CAD build for the part. Positions are in the model's coordinates, mm. Face numbers are marked on the shaded views. Coordinates: 2 decimals unless noted, no trailing zeros. Order: outer loops, then holes, each group sorted by start corner. A loop starts at its lowest first (then second) coordinate and runs counter-clockwise, first axis right, second up. Notation, with made-up numbers: M 3,23.5 L 35,23.5 A32 ccw 35,50.5 Z; hole C 77,42 d8. An arc over 180 degrees is marked long. Write item = value, one per line.
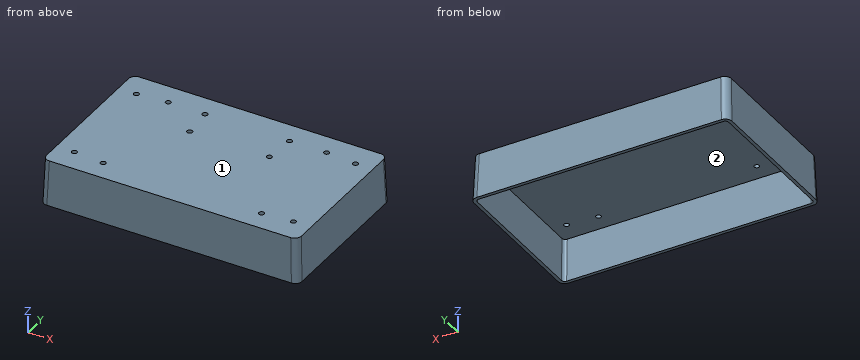
from build123d import *

# Parameters (mm, degrees)
SKETCH_1_W      = 148
SKETCH_1_H      = 88
SKETCH_1_R      = 1.5
EXTRUDE_1_DEPTH = 25
EXTRUDE_1_DRAFT = 2
FILLET_1_R      = 2
SHELL_1_T       = 2


with BuildPart() as part:
    # Эскиз1 → Бобышка-Вытянуть1 (with draft: the straight prism first)
    with BuildSketch(Plane.XY):
        with Locations((-40.018678, 18.487832)):
            Rectangle(SKETCH_1_W, SKETCH_1_H)
        with Locations((7.364962, 51.289097)):
            Circle(SKETCH_1_R, mode=Mode.SUBTRACT)
        with Locations((25.491262, 49.776217)):
            Circle(SKETCH_1_R, mode=Mode.SUBTRACT)
        with Locations((25.471663, -13.623467)):
            Circle(SKETCH_1_R, mode=Mode.SUBTRACT)
        with Locations((7.364962, -15.128048)):
            Circle(SKETCH_1_R, mode=Mode.SUBTRACT)
        with Locations((-14.633582, 51.078679)):
            Circle(SKETCH_1_R, mode=Mode.SUBTRACT)
        with Locations((-16.116192, 32.998149)):
            Circle(SKETCH_1_R, mode=Mode.SUBTRACT)
        with Locations((-65.018894, 51.078679)):
            Circle(SKETCH_1_R, mode=Mode.SUBTRACT)
        with Locations((-63.53497, 32.998149)):
            Circle(SKETCH_1_R, mode=Mode.SUBTRACT)
        with Locations((-87.0372, 51.289097)):
            Circle(SKETCH_1_R, mode=Mode.SUBTRACT)
        with Locations((-105.122155, 49.776217)):
            Circle(SKETCH_1_R, mode=Mode.SUBTRACT)
        with Locations((-87.0372, -15.128048)):
            Circle(SKETCH_1_R, mode=Mode.SUBTRACT)
        with Locations((-105.094004, -13.623467)):
            Circle(SKETCH_1_R, mode=Mode.SUBTRACT)
    extrude(amount=-EXTRUDE_1_DEPTH)
    # Бобышка-Вытянуть1: the draft: its side faces are tilted about the plane it starts from
    extrude_1_sides = [part.faces().sort_by_distance(p)[0] for p in [
        (-40.018678, 62.487832, -12.5),
        (-114.018678, 18.487832, -12.5),
        (-40.018678, -25.512168, -12.5),
        (33.981322, 18.487832, -12.5),
        (5.864962, 51.289097, -12.5),
        (23.991262, 49.776217, -12.5),
        (23.971663, -13.623467, -12.5),
        (5.864962, -15.128048, -12.5),
        (-16.133582, 51.078679, -12.5),
        (-17.616192, 32.998149, -12.5),
        (-66.518894, 51.078679, -12.5),
        (-65.03497, 32.998149, -12.5),
        (-88.5372, 51.289097, -12.5),
        (-106.622155, 49.776217, -12.5),
        (-88.5372, -15.128048, -12.5),
        (-106.594004, -13.623467, -12.5),
    ]]
    draft(extrude_1_sides, Plane.XY, EXTRUDE_1_DRAFT)

    # Скругление1
    fillet_1_edges = [part.edges().sort_by_distance(p)[0] for p in [
        (34.417831, -25.948678, -12.5),
        (-114.455188, -25.948678, -12.5),
        (-114.455188, 62.924342, -12.5),
        (34.417831, 62.924342, -12.5),
    ]]
    fillet(fillet_1_edges, radius=FILLET_1_R)

    # Оболочка1
    shell_1_openings = [part.faces().sort_by_distance(p)[0] for p in [
        (-40.018892, 18.479465, -25),
        (6.301471, 51.289097, -12.5),
        (24.427772, 49.776217, -12.5),
        (24.408173, -13.623467, -12.5),
        (6.301471, -15.128048, -12.5),
        (-15.697073, 51.078679, -12.5),
        (-17.179682, 32.998149, -12.5),
        (-66.082384, 51.078679, -12.5),
        (-64.59846, 32.998149, -12.5),
        (-88.10069, 51.289097, -12.5),
        (-106.185646, 49.776217, -12.5),
        (-88.10069, -15.128048, -12.5),
        (-106.157495, -13.623467, -12.5),
    ]]
    offset(amount=SHELL_1_T, openings=shell_1_openings, kind=Kind.INTERSECTION)


solid = part.part
(1) Slice it at B-B, the plane y = 2. Write the cut outline in (x, z).
Evaluation:
outline = M -116.89,-25 L -114.89,-25 L -114.02,0 L 33.98,0 L 34.85,-25 L 36.86,-25 L 35.91,2 L -115.95,2 Z
(2) Wall check: line 1 (Z direction, x = 9.5, y = 41.5); line 2 (Y direction, x = -67.5, z = -14.75); line 3 (X direction, y = 27, z = -22.5). Give the ranges that are in metal, low to high. Write a range as from..to.
Evaluation:
line_1 = 0..2
line_2 = -28.03..-26.03, 63..65
line_3 = -116.81..-114.8, 34.77..36.77
(3) Slice it at A-A, the plane x = -37.5. Write the cut outline in (y, z), then the cut area to 3 significant figures.
Evaluation:
outline = M -28.39,-25 L -26.39,-25 L -25.51,0 L 62.49,0 L 63.36,-25 L 65.36,-25 L 64.42,2 L -27.44,2 Z
area = 284 mm²
(4) Pull direction X, two halves, no side cores. Call the marked faces 1 and 2: +X half, -X half, draft (parallel to the pull), parting line (faces both ways), or undercut.
Evaluation:
face_1 = draft
face_2 = undercut
(5) Pin check, flat tips, straight feed: pin 1 Ø12 at (x, z) = (-48, -1.5) entering from -Y; pin 2 Ø3 at (y, z) = (21.5, -15.5) entering from +X; pin 3 Ø1.5 at (y, z) = (16, -13) entering from +X. Stop position of each tip, or through.
Evaluation:
pin_1 = -27.78
pin_2 = 36.58
pin_3 = 36.46
